```python
from build123d import *

# Parameters (mm, degrees)
BOSS_EXTRUDE1_DEPTH                               = 1
BOSS_EXTRUDE1_DEPTH_BACK                          = 1
SKETCH2_W                                         = 1
SKETCH2_H                                         = 5
BOSS_EXTRUDE3_DEPTH                               = 1
FILLET1_R                                         = 2
FILLET2_R                                         = 0.5
CSK_FOR_1_FLAT_HEAD_MACHINE_SCREW_100_D           = 2.0574
CSK_FOR_1_FLAT_HEAD_MACHINE_SCREW_100_DEPTH       = 5.381894681
CSK_FOR_1_FLAT_HEAD_MACHINE_SCREW_100_CSINK_D     = 3.7084
CSK_FOR_1_FLAT_HEAD_MACHINE_SCREW_100_CSINK_ANGLE = 100
CSK_FOR_1_FLAT_HEAD_MACHINE_SCREW_100_TIP         = 0.618105319


with BuildPart() as part:
    # Sketch1 → Boss-Extrude1 (new, two sides: drawn at the far end of the back side and taken through both)
    with BuildSketch(Plane.XY.offset(-BOSS_EXTRUDE1_DEPTH_BACK)):
        with BuildLine():
            Line((-70.765177629, -17.59), (-51.765177629, -17.59))
            Line((-51.765177629, -17.59), (-51.765177629, -47.59))
            Line((-51.765177629, -47.59), (-70.765177629, -47.59))
            Line((-70.765177629, -47.59), (-70.765177629, -35.59))
            ThreePointArc((-70.765177629, -35.59), (-74.265177629, -32.09), (-70.765177629, -28.59))
            Line((-70.765177629, -28.59), (-70.765177629, -17.59))
        make_face()
    extrude(amount=BOSS_EXTRUDE1_DEPTH + BOSS_EXTRUDE1_DEPTH_BACK)

    # Sketch2 → Boss-Extrude3 (add)
    with BuildSketch(Plane.XY.offset(1)):
        with Locations((-51.265177629, -32.59)):
            Rectangle(SKETCH2_W, SKETCH2_H)
    extrude(amount=-BOSS_EXTRUDE3_DEPTH)

    # Fillet1
    fillet1_edges = [part.edges().sort_by_distance(p)[0] for p in [
        (-70.765177629, -17.59, 0),
        (-51.765177629, -17.59, 0),
        (-51.765177629, -47.59, 0),
        (-70.765177629, -47.59, 0),
    ]]
    fillet(fillet1_edges, radius=FILLET1_R)

    # Fillet2
    fillet2_edges = [part.edges().sort_by_distance(p)[0] for p in [
        (-50.765177629, -30.09, 0.5),
        (-50.765177629, -35.09, 0.5),
    ]]
    fillet(fillet2_edges, radius=FILLET2_R)

    # CSK for #1 Flat Head Machine Screw (100)1
    with Locations(Plane(origin=(-71.606429364, -32.068746038, -1), x_dir=(-1, 0, 0), z_dir=(0, 0, -1))):
        with Locations((0, 0)):
            CounterSinkHole(CSK_FOR_1_FLAT_HEAD_MACHINE_SCREW_100_D / 2, CSK_FOR_1_FLAT_HEAD_MACHINE_SCREW_100_CSINK_D / 2, depth=CSK_FOR_1_FLAT_HEAD_MACHINE_SCREW_100_DEPTH, counter_sink_angle=CSK_FOR_1_FLAT_HEAD_MACHINE_SCREW_100_CSINK_ANGLE)
            with Locations((0, 0, -(CSK_FOR_1_FLAT_HEAD_MACHINE_SCREW_100_DEPTH + CSK_FOR_1_FLAT_HEAD_MACHINE_SCREW_100_TIP / 2))):  # 118° drill point
                Cone(0, CSK_FOR_1_FLAT_HEAD_MACHINE_SCREW_100_D / 2, CSK_FOR_1_FLAT_HEAD_MACHINE_SCREW_100_TIP, mode=Mode.SUBTRACT)


solid = part.part
```
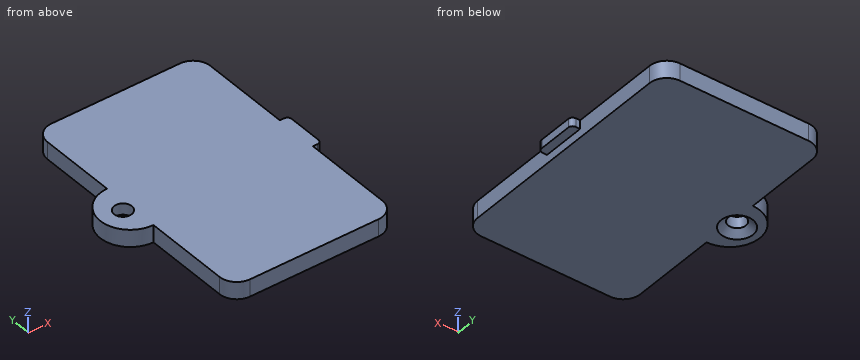
Geometry: final body of the model. Coordinates: model frame, mm. Coordinates: 2 decimals unless noted, no trailing zeros. Order: outer loops, then holes, each group sorted by start corner. A loop starts at its lowest first (then second) coordinate and runs counter-clockwise, first axis right, second up. Notation, with made-up numbers: M 2.5,38.25 L 43.5,38.25 A17 cw 43.5,68.25 Z; hole C 18,59.25 d1. An arc over 180 degrees is marked long. Answer in a Markdown table with one row per item. Add a question column.
Q1. Section query A-A on z = 0.35. Return the cut outline in (x, y).
Q2. Section query B-B on y = -24.5. Return the cut outline in (x, z).
Q3. Line query: L1, parallel to X at y = -44.5, z = 0.2; L2, parallel to Y at x = -72, z = -0.9; L3, parallel to Y at x = -52.5, z = 0.95. Output: solid intervals per line, ascending.
Q4. Contact query for flat-ended pins moving along their axis: P1, Ø1, axis at y = -41, z = 0.5, coming from the -X side; P2, Ø2.5, axis at x = -71.61, y = -32.07, coming from the +Z side; P3, Ø0.8, axis at x = -51, y = -32.5, coming from the -Z side. Output: stop coordinate, or through.
Completed:
| question | item | result |
|---|---|---|
| 1 | outline | M -70.77,-45.59 A2 ccw -68.77,-47.59 L -53.77,-47.59 A2 ccw -51.77,-45.59 L -51.77,-35.09 L -51.27,-35.09 A0.5 ccw -50.77,-34.59 L -50.77,-30.59 A0.5 ccw -51.27,-30.09 L -51.77,-30.09 L -51.77,-19.59 A2 ccw -53.77,-17.59 L -68.77,-17.59 A2 ccw -70.77,-19.59 L -70.77,-28.59 A3.5 ccw -70.77,-35.59 Z; hole C -71.61,-32.07 d2.06 |
| 2 | outline | M -70.77,-1 L -51.77,-1 L -51.77,1 L -70.77,1 Z |
| 3 | L1 | x = -70.77 to -51.77 |
| 3 | L2 | y = -35.36 to -33.76, -30.38 to -28.82 |
| 3 | L3 | y = -47.14 to -18.04 |
| 4 | P1 | stops at x = -70.77 |
| 4 | P2 | stops at z = 1 |
| 4 | P3 | stops at z = 0 |
